from build123d import *

# Parameters (mm, degrees)
ESQUISSE1_R        = 4.5
ESQUISSE1_R_2      = 5.5
BOSS_EXTRU_1_DEPTH = 11
ESQUISSE3_R        = 9.5
ESQUISSE3_R_2      = 4.5
BOSS_EXTRU_3_DEPTH = 6


with BuildPart() as part:
    # Esquisse1 → Boss.-Extru.1 (new body)
    with BuildSketch(Plane(origin=(0, 0, 0), x_dir=(1, 0, 0), z_dir=(0, 1, 0))):
        with BuildLine():
            Line((-28.930476165, 16.379180347), (-6.847605923, -6.584853311))
            ThreePointArc((-6.847605923, -6.584853311), (8.382701799, -4.469934065), (1.652173913, 9.355229626))
            ThreePointArc((1.652173913, 9.355229626), (0.467738245, 10.039382479), (0, 11.324751653))
            Line((0, 11.324751653), (0, 50.675248347))
            ThreePointArc((0, 50.675248347), (0.467738245, 51.960617521), (1.652173913, 52.644770374))
            ThreePointArc((1.652173913, 52.644770374), (8.967130897, 58.863032758), (7.12365328, 68.285186071))
            Line((7.12365328, 68.285186071), (-10.547240372, 88.313442691))
            ThreePointArc((-10.547240372, 88.313442691), (-31.313992211, 85.185213109), (-19.920468372, 67.543461019))
            Line((-19.920468372, 67.543461019), (-14, 67.543461019))
            ThreePointArc((-14, 67.543461019), (-12.585786438, 66.957674582), (-12, 65.543461019))
            Line((-12, 65.543461019), (-12, 39.543461019))
            ThreePointArc((-12, 39.543461019), (-12.585786438, 38.129247457), (-14, 37.543461019))
            Line((-14, 37.543461019), (-19.920468372, 37.543461019))
            ThreePointArc((-19.920468372, 37.543461019), (-31.42163154, 29.939709154), (-28.930476165, 16.379180347))
        make_face()
        with Locations(Location((0, 0, 0), (0, 0, 270))):  # turned: the seam where the file's is
            Circle(ESQUISSE1_R, mode=Mode.SUBTRACT)
        with Locations(Location((-19.920468372, 25.043461019, 0), (0, 0, 270))):  # turned: the seam where the file's is
            Circle(ESQUISSE1_R_2, mode=Mode.SUBTRACT)
        with Locations(Location((0, 62, 0), (0, 0, 270))):  # turned: the seam where the file's is
            Circle(ESQUISSE1_R, mode=Mode.SUBTRACT)
        with Locations(Location((-19.920468372, 80.043461019, 0), (0, 0, 270))):  # turned: the seam where the file's is
            Circle(ESQUISSE1_R_2, mode=Mode.SUBTRACT)
    extrude(amount=BOSS_EXTRU_1_DEPTH)

    # Esquisse3 → Boss.-Extru.3 (add)
    with BuildSketch(Plane(origin=(0, 11, 0), x_dir=(1, 0, 0), z_dir=(0, 1, 0))):
        with Locations(Location((0, 0, 0), (0, 0, 79.984589832))):  # turned: the seam where the file's is
            Circle(ESQUISSE3_R)
        with Locations(Location((0, 0, 0), (0, 0, 270))):  # turned: the seam where the file's is
            Circle(ESQUISSE3_R_2, mode=Mode.SUBTRACT)
        with Locations(Location((0, 62, 0), (0, 0, 41.421900303))):  # turned: the seam where the file's is
            Circle(ESQUISSE3_R)
        with Locations(Location((0, 62, 0), (0, 0, 270))):  # turned: the seam where the file's is
            Circle(ESQUISSE3_R_2, mode=Mode.SUBTRACT)
    extrude(amount=BOSS_EXTRU_3_DEPTH)


solid = part.part
Design review of the part built by this model. Coordinates are the model's own, in mm. A direction names the side the tool comes from. Coordinates: 2 decimals unless noted, no trailing zeros. Order: outer loops, then holes, each group sorted by start corner. A loop starts at its lowest first (then second) coordinate and runs counter-clockwise, first axis right, second up.
Item 1: For line 1 (X direction, y = 8.25, z = -50); line 2 (Z direction, x = 8, y = 4.75); line 3 (Z direction, x = -1, y = 8.75), list the stretches that pass through material, from the lowest coordinate up.
Item 2: The part is to be moulded in two halves that separate along X. For faces 1 (the cylindrical face through (0.5, 5.4, -10)), 2 (the cylindrical face through (-12.6, 5.42, -66.97)), 3 (the cylindrical face through (1.352, 8.381, -57.708)), 4 (the flat face through (-11.8, 0, -42.2)), say which applies: pulls with the +X half, pulls with the -X half, needs draft (parallel to the pull), parting line crosses it, or undercut.
Item 3: Take a section at D-D, the plane y = 13. Write out the cut boundary in (x, z), then the cut area to 3 significant figures.
Item 4: For pin 1 Ø1.8 at (x, y) = (-17.5, 3) entering from -Z; pin 2 Ø11.5 at (x, z) = (0, 0) entering from -Y; pin 3 Ø10 at (y, z) = (14.5, -43) entering from +X; pin 4 Ø6 at (y, z) = (3, -5.5) entering from -X, all flat-tipped, find the tip position at first contact; note any pin that passes through.
Item 5: Take a section at C-C, the plane x = -16. Write out the cut boundary in (y, z), then the cut area to 3 significant figures.
Item 6: Take a section at A-A, the plane z = -62. Write out the cut boundary in (x, y), then the cut area to 4 significant figures.
Item 7: For faces 5 (the flat face through (-12, 5, -53)), 6 (the flat face through (1.6, 17, -66.4)), 7 (the cylindrical face through (0.46, 5.42, -51.95)), list the 3-axis set-ups (+Z, -Z, +X, -X, +Y, -Y) from which the entire face can be reached by the end or side of a thin tool; tool diameter is ignored.
Item 8: Take a section at B-B, the plane y = 4. Write out the cut boundary in (x, z).
The answers:
1. line 1: x = -12 to 0
1. line 2: z = -67.12 to -56.88, -5.12 to 5.12
1. line 3: z = -77.49 to -66.39, -57.61 to -4.39, 4.39 to 9.45
2. face 1: pulls with the +X half
2. face 2: pulls with the -X half
2. face 3: undercut
2. face 4: needs draft
3. outline: circle Ø19 at (0, -62); circle Ø19 at (0, 0); hole circle Ø9 at (0, -62); hole circle Ø9 at (0, 0)
3. area: 440 mm2
4. pin 1: stops at z = -92.45
4. pin 2: stops at y = 0
4. pin 3: stops at x = 0
4. pin 4: stops at x = -21.35
5. outline: (0, -91.91) - (11, -91.91) - (11, -83.9) - (0, -83.9) - close; (0, -76.19) - (11, -76.19) - (11, -67.54) - (0, -67.54) - close; (0, -37.54) - (11, -37.54) - (11, -28.9) - (0, -28.9) - close; (0, -21.19) - (11, -21.19) - (11, -2.93) - (0, -2.93) - close
5. area: 479 mm2
6. outline: (-12, 0) - (-4.5, 0) - (-4.5, 17) - (-9.5, 17) - (-9.5, 11) - (-12, 11) - close; (4.5, 0) - (9.5, 0) - (9.5, 17) - (4.5, 17) - close
6. area: 197.5 mm2
7. face 5: -X, +Y, -Y
7. face 6: +Z, -Z, +X, -X, +Y
7. face 7: +X, +Y, -Y
8. outline: (-28.93, -16.38) arc R12.5 ccw to (-19.92, -37.54) - (-14, -37.54) arc R2 cw to (-12, -39.54) - (-12, -65.54) arc R2 cw to (-14, -67.54) - (-19.92, -67.54) arc R12.5 ccw (long way) to (-10.55, -88.31) - (7.12, -68.29) arc R9.5 ccw to (1.65, -52.64) arc R2 cw to (0, -50.68) - (0, -11.32) arc R2 cw to (1.65, -9.36) arc R9.5 ccw (long way) to (-6.85, 6.58) - close; hole circle Ø11 at (-19.92, -80.04); hole circle Ø11 at (-19.92, -25.04); hole circle Ø9 at (0, -62); hole circle Ø9 at (0, 0)
